Work out the finished part from the listing and answer in its coordinate system (mm). A direction names the side the tool comes from. Give positions to 0.01 mm unless a question says otherwise; leave off trailing zeros. Loops run counter-clockwise (first coordinate to the right, second up) from the corner with the lowest first, then second, coordinate; pieces in that order, holes last. Notation, with made-up numbers: (63, 82.5) - (81, 82.5) arc R9 ccw to (81, 86.5) - close; hole circle Ø1 at (31, -25). An arc over 180 degrees is marked (long way). One line per question, with ' | ' between items.
Autodesk Fusion 360 part; units mm, degrees
sketch "Sketch1" plane through (0, 0, 0) normal (0, 0, 1) x (1, 0, 0)
  line L0 (0, 0) -> (22, 0)
  circle A0 centre (22, 0) radius 2.5
  line L1 (22, 0) -> (14, 0)
  circle A1 centre (14, 0) radius 2.5
  circle A2 centre (0, 0) radius 2.4
  line L2 (22.01, -4) -> (-0.01, -4)
  line L3 (-4, -0.01) -> (-4, 0.01)
  line L4 (-0.01, 4) -> (22.01, 4)
  line L5 (26, 0.01) -> (26, -0.01)
  arc A3 (-4, -0.01) -> (-0.01, -4) centre (-0.01, -0.01) ccw
  arc A4 (-0.01, 4) -> (-4, 0.01) centre (-0.01, 0.01) ccw
  arc A5 (26, 0.01) -> (22.01, 4) centre (22.01, 0.01) ccw
  arc A6 (22.01, -4) -> (26, -0.01) centre (22.01, -0.01) ccw
  dimension "d1" = 22
  dimension "d2" = 5
  dimension "d3" = 8
  dimension "d4" = 5
  dimension "d5" = 4.8
  dimension "d6" = 3.99
  dimension "d7" = 3.99
  dimension "d8" = 3.99
  dimension "d9" = 3.99
extrude "Extrude1" add sketch "Sketch1" along normal blind 7.5 contours A2 | L2 L3 L4 L5 A3 A4 A5 A6
extrude "Extrude2" cut sketch "Sketch1" along normal blind 2.5 contours A2
sketch "Sketch2" plane through (0, 0, 7.5) normal (0, 0, 1) x (-1, 0, 0)
  circle A0 centre (-22, 0) radius 2.5
  circle A1 centre (-14, 0) radius 2.5
  arc A2 (4, 0.01) -> (0.01, 4) centre (0.01, 0.01) ccw
  line L0 (0.01, 4) -> (-22.01, 4)
  arc A3 (-22.01, 4) -> (-26, 0.01) centre (-22.01, 0.01) ccw
  line L1 (-26, 0.01) -> (-26, -0.01)
  arc A4 (-26, -0.01) -> (-22.01, -4) centre (-22.01, -0.01) ccw
  line L2 (-22.01, -4) -> (0.01, -4)
  arc A5 (0.01, -4) -> (4, -0.01) centre (0.01, -0.01) ccw
  line L3 (4, -0.01) -> (4, 0.01)
  circle A6 centre (0.01, -0.01) radius 1.25
  dimension "d14" = 2.5
extrude "Extrude3" cut sketch "Sketch2" against normal blind 100 contours A6
sketch "Sketch3" plane through (0, 0, 7.5) normal (0, 0, 1) x (-1, 0, 0)
  circle A0 centre (0, 0) radius 2.5
  dimension "d17" = 5
extrude "Extrude4" cut sketch "Sketch3" against normal blind 3
sketch "Sketch4" plane through (0, 0, 0) normal (0, 0, 1) x (1, 0, 0)
  circle A0 centre (14, 0) radius 3
  circle A1 centre (22, 0) radius 3
  dimension "d20" = 6
  dimension "d21" = 6
extrude "Extrude5" cut sketch "Sketch4" along normal blind 1 contours A0
extrude "Extrude6" cut sketch "Sketch4" along normal blind 1 contours A1
sketch "Sketch5" plane through (0, 0, 7.5) normal (0, 0, 1) x (-1, 0, 0)
  circle A0 centre (0, 0) radius 2.5
  circle A1 centre (-22, 0) radius 2.5
  circle A2 centre (-14, 0) radius 2.5
  arc A3 (4, 0.01) -> (0.01, 4) centre (0.01, 0.01) ccw
  line L0 (0.01, 4) -> (-22.01, 4)
  arc A4 (-22.01, 4) -> (-26, 0.01) centre (-22.01, 0.01) ccw
  line L1 (-26, 0.01) -> (-26, -0.01)
  arc A5 (-26, -0.01) -> (-22.01, -4) centre (-22.01, -0.01) ccw
  line L2 (-22.01, -4) -> (0.01, -4)
  arc A6 (0.01, -4) -> (4, -0.01) centre (0.01, -0.01) ccw
  line L3 (4, -0.01) -> (4, 0.01)
  circle A7 centre (-14, 0) radius 3
  circle A8 centre (-22.01, -0.01) radius 3
  dimension "d26" = 6
  dimension "d27" = 6
extrude "Extrude7" cut sketch "Sketch5" against normal blind 1 contours A8
extrude "Extrude8" cut sketch "Sketch5" against normal blind 1 contours A7
1. Which of the six approach directions +Z, -Z, +X, -X, +Y, -Y give full straight-line access (tool end or side, diameter ignored) to faces 1 (the flat face through (16, -2, 6.5)), 2 (the cylindrical face through (19, -0.1, 0.5)), 3 (the cylindrical face through (-2.86, 2.8, 3.7))?
Evaluation:
face 1: +Z | face 2: -Z | face 3: +Z, -Z, -X, +Y
2. Consider L1, parallel to X at y = 0.01, z = 3.55; L2, parallel to X at y = 0.01, z = 7; L3, parallel to Y at x = 14, z = 3.45. Determine where each line is inside the solid, lowest interval first.
Evaluation:
L1: -4 to -1.26, 1.24 to 11.5, 16.5 to 19.5, 24.5 to 26 | L2: -4 to -2.5, 2.5 to 11, 17 to 19.01, 25.01 to 26 | L3: -4 to -2.5, 2.5 to 4
3. Find section B-B on x = 14. Write down the section's boundary in (y, z), then the cut area to 3 significant figures.
Evaluation:
outline: (-4, 0) - (-3, 0) - (-3, 1) - (-2.5, 1) - (-2.5, 6.5) - (-3, 6.5) - (-3, 7.5) - (-4, 7.5) - close; (2.5, 1) - (3, 1) - (3, 0) - (4, 0) - (4, 7.5) - (3, 7.5) - (3, 6.5) - (2.5, 6.5) - close | area: 20.5 mm2
4. Flat-ended cylindrical pins translate along their axes: pin 1 (3 mm diameter, centred on x = 23, y = 0.5, fed in from -Z); pin 2 (4.5 mm diameter, centred on x = 0, y = 0, fed in from +Z); pin 3 (1.4 mm diameter, centred on x = 0, y = 1, fed in from -Z). Find the tip coordinate at first contact, or state that the pin passes through.
Evaluation:
pin 1: z = 1 | pin 2: z = 4.5 | pin 3: z = 2.5
5. Determine the mould class of faces 4 (the flat face through (11, 4, 4)), 5 (the cylindrical face through (1.29, -2.024, 1.232)), 6 (the cylindrical face through (11, -0.1, 0.5)), 7 (the cylindrical face through (24.86, -2.8, 3.7)) for opening direction X: +X half, -X half, draft (parallel to the pull), parting line (faces both ways), or undercut.
Evaluation:
face 4: draft | face 5: undercut | face 6: undercut | face 7: +X half
6. Find section A-A on z = 6. State how many separate pieces and enclosed holes the cut face has, then the cut area to 3 significant figures.
Evaluation:
separate pieces: 1 | enclosed holes: 3 | area: 167 mm2
7. Find section C-C on x = 22.5. Write down the section's boundary in (y, z), then the cut area to 3 significant figures.
Evaluation:
outline: (-3.97, 0) - (-2.96, 0) - (-2.96, 1) - (-2.45, 1) - (-2.45, 6.5) - (-2.95, 6.5) - (-2.95, 7.5) - (-3.97, 7.5) - close; (2.45, 1) - (2.96, 1) - (2.96, 0) - (3.97, 0) - (3.97, 7.5) - (2.97, 7.5) - (2.97, 6.5) - (2.45, 6.5) - close | area: 20.8 mm2
